Autodesk Inventor part; units mm, degrees
ref_plane "YZ Plane" through (0, 0, 0) normal (1, 0, 0) x (0, 1, 0)
ref_plane "XZ Plane" through (0, 0, 0) normal (0, 1, 0) x (-1, 0, 0)
ref_plane "XY Plane" through (0, 0, 0) normal (0, 0, 1) x (1, 0, 0)
sketch "Sketch1" plane through (0, 0, 0) normal (0, 0, 1) x (1, 0, 0)
  line L0 (-110, 22.5) -> (110, 22.5)
  line L1 (110, 22.5) -> (110, -22.5)
  line L2 (110, -22.5) -> (-110, -22.5)
  line L3 (-110, -22.5) -> (-110, 22.5)
  point P0 (0, 0)
  point P1 (110, 0)
  point P2 (0, 22.5)
  dimension "d0" = 220
  dimension "d1" = 45
extrude "Extrusion1" add sketch "Sketch1" along normal blind 15
sketch "Sketch2" plane through (0, 0, 15) normal (0, 0, 1) x (1, 0, 0)
  line L0 (-105, 15) -> (-55, 15) construction
  line L1 (-105, 12.5) -> (-55, 12.5)
  line L2 (-55, 17.5) -> (-105, 17.5)
  arc A0 (-105, 17.5) -> (-105, 12.5) centre (-105, 15) ccw
  arc A1 (-55, 12.5) -> (-55, 17.5) centre (-55, 15) ccw
  line L3 (-105, -15) -> (-55, -15) construction
  line L4 (-105, -17.5) -> (-55, -17.5)
  line L5 (-55, -12.5) -> (-105, -12.5)
  arc A2 (-105, -12.5) -> (-105, -17.5) centre (-105, -15) ccw
  arc A3 (-55, -17.5) -> (-55, -12.5) centre (-55, -15) ccw
  line L6 (-80, 15) -> (-80, -15) construction
  line L7 (-110, 22.5) -> (-110, -22.5)
  point P0 (0, 0)
  point P1 (-80, 0)
  dimension "d4" = 5
  dimension "d5" = 30
  dimension "d6" = 50
  dimension "d7" = 5
extrude "Extrusion2" cut sketch "Sketch2" against normal through all
mirror "Mirror1" about plane through (0, 0, 0) normal (1, 0, 0) of "Extrusion2"
fillet "Fillet1" radius 2 4 edges at (-110, -22.5, 7.5) (-110, 22.5, 7.5) (110, 22.5, 7.5) (110, -22.5, 7.5)
chamfer "Chamfer1" distance 0.5 angle 45 16 edges at (0, 22.5, 15) (-109.4142, 21.9142, 15) (-110, 0, 15) (-109.4142, -21.9142, 15) (0, -22.5, 15) (109.4142, -21.9142, 15) (110, 0, 15) (109.4142, 21.9142, 15) (0, -22.5, 0) (109.4142, -21.9142, 0) (110, 0, 0) (109.4142, 21.9142, 0) (0, 22.5, 0) (-109.4142, 21.9142, 0) (-110, 0, 0) (-109.4142, -21.9142, 0)
sketch "Sketch3" plane through (0, 0, 15) normal (0, 0, -1) x (-1, 0, 0)
  line L0 (-20, 0) -> (20, 0) construction
  point P0 (0, 0)
  point P1 (0, 0)
  dimension "d14" = 40
hole "Hole1" at (20, 0, 15) at (-20, 0, 15) direction (0, 0, -1) diameter 6 end through all counterbore diameter 12 counterbore depth 5
properties part number "clamp-foot" material "Aluminum 6061"
The listing builds one solid part. Answer for the finished solid, in the listing's coordinates (mm). A direction names the side the tool comes from. Give positions to 0.01 mm unless a question says otherwise; leave off trailing zeros. Order: outer loops, then holes, each group sorted by start corner. A loop starts at its lowest first (then second) coordinate and runs counter-clockwise, first axis right, second up. Notation, with made-up numbers: (88.5, 61.5) - (95.5, 61.5) arc R14 cw to (95.5, 85.5) - close; hole circle Ø2 at (70.25, 26). An arc over 180 degrees is marked (long way). Answer in a Markdown table with one row per item. Add a question column.
Q1. The part is cut by section C-C (z = 3.75). Determine the outline of the cut face in (x, y), then the cut area to 3 significant figures.
Q2. Find the intervals of material crossed by line 1 along X through (y, z) = (0, 5.25); line 2 along X through (y, z) = (0, 13.2); line 3 along Y through (x, z) = (20, 4.75), in increasing order. Write a range as [from, to].
Q3. Which of the six approach directions +Z, -Z, +X, -X, +Y, -Y give full straight-line access (tool end or side, diameter ignored) to faces 4 (the flat face through (-2, 0, 15)), 5 (the flat face through (-80, -17.5, 8)), 6 (the cylindrical face through (14.05, 0.78, 12.46))?
Q4. Given P1, Ø7, axis at x = 20, y = 0, coming from the +Z side, flat-ended and moving along its own axis, determine where the tip first touches the part or whether it passes through.
Q5. The part is cut by section A-A (x = 20). Determine the outline of the cut face in (y, z), then the cut area to 4 significant figures.
Q6. The part is cut by section D-D (y = -15). Determine the outline of the cut face in (x, z).
Q7. For a pull along X with two mould halves and no side action, classify faces 1 (the flat face through (110, 0, 7)), 2 (the flat face through (-80, 17.5, 8)), 3 (the flat face through (-2, 22.5, 7)) as released by +X, released by -X, zero draft, split by the parting line, or undercut.
Q8. The part is cut by section B-B (y = 0). Determine the outline of the cut face in (x, z).
Determined:
| question | item | result |
|---|---|---|
| 1 | outline | (-110, -20.5) arc R2 ccw to (-108, -22.5) - (108, -22.5) arc R2 ccw to (110, -20.5) - (110, 20.5) arc R2 ccw to (108, 22.5) - (-108, 22.5) arc R2 ccw to (-110, 20.5) - close; hole (-105, -17.5) - (-55, -17.5) arc R2.5 ccw to (-55, -12.5) - (-105, -12.5) arc R2.5 ccw to start; hole (-105, 12.5) - (-55, 12.5) arc R2.5 ccw to (-55, 17.5) - (-105, 17.5) arc R2.5 ccw to start; hole circle Ø6 at (-20, 0); hole circle Ø6 at (20, 0); hole (55, -17.5) - (105, -17.5) arc R2.5 ccw to (105, -12.5) - (55, -12.5) arc R2.5 ccw to start; hole (55, 12.5) - (105, 12.5) arc R2.5 ccw to (105, 17.5) - (55, 17.5) arc R2.5 ccw to start |
| 1 | area | 8,760 mm² |
| 2 | line 1 | x = [-110, -23], [-17, 17], [23, 110] |
| 2 | line 2 | x = [-110, -26], [-14, 14], [26, 110] |
| 2 | line 3 | y = [-22.5, -3], [3, 22.5] |
| 3 | face 4 | +Z, +X, -X, +Y, -Y |
| 3 | face 5 | +Z, -Z |
| 3 | face 6 | +Z |
| 4 | P1 | stops at z = 10 |
| 5 | outline | (-22.5, 0.5) - (-22, 0) - (-3, 0) - (-3, 10) - (-6, 10) - (-6, 15) - (-22, 15) - (-22.5, 14.5) - close; (3, 0) - (22, 0) - (22.5, 0.5) - (22.5, 14.5) - (22, 15) - (6, 15) - (6, 10) - (3, 10) - close |
| 5 | area | 554.5 mm² |
| 6 | outline | (-110, 0.5) - (-109.5, 0) - (-107.5, 0) - (-107.5, 15) - (-109.5, 15) - (-110, 14.5) - close; (-52.5, 0) - (52.5, 0) - (52.5, 15) - (-52.5, 15) - close; (107.5, 0) - (109.5, 0) - (110, 0.5) - (110, 14.5) - (109.5, 15) - (107.5, 15) - close |
| 7 | face 1 | released by +X |
| 7 | face 2 | undercut |
| 7 | face 3 | zero draft |
| 8 | outline | (-110, 0.5) - (-109.5, 0) - (-23, 0) - (-23, 10) - (-26, 10) - (-26, 15) - (-109.5, 15) - (-110, 14.5) - close; (-17, 0) - (17, 0) - (17, 10) - (14, 10) - (14, 15) - (-14, 15) - (-14, 10) - (-17, 10) - close; (23, 0) - (109.5, 0) - (110, 0.5) - (110, 14.5) - (109.5, 15) - (26, 15) - (26, 10) - (23, 10) - close |
